Answer from the drawing. Dimensions are ordinates in mm from the lowest x, y and z of the part. A direction names the side the tool comes from. Round coordinates to 2 decimals unless told otherwise and drop trailing zeros. Write each loop counter-clockwise with the first axis right and the second up, starting at its lowest first coordinate (ties: lowest second). Pieces come first, ordered by that corner, then holes.
1. Find section A-A (y = 62). Write down the section's boundary in (x, z).
2. Find section C-C (z = 1.25). Write down the section's boundary in (x, y).
3. Find section D-D (x = 37). Write down the section's boundary in (y, z), and give its area (3 significant figures).
4. Flat-ended cylindrical pins translate along their axes: pin 1 Ø4 at (x, z) = (12.5, 4) entering from +Y (1 decimal); pin 2 Ø6 at (y, z) = (20.5, 8.5) entering from +X; pin 3 Ø2.5 at (x, y) = (46.9, 71.9) entering from -Z; pin 4 Ø5 at (x, z) = (4, 4) entering from +Y. Find the tip coordinate at first contact, or state that the pin passes through.
5. Find section B-B (x = 6). Write down the section's boundary in (y, z).
6. Straight lines are drawn through the part: probe 1 along X at (y, z) = (62.5, 4.75); probe 2 along Y at (x, z) = (37, 6.5); probe 3 along Y at (x, z) = (37, 2.05). For each, find the intervals that lie inside material, in ascending order.
7. A tool of negligible diameter and unlimited length cuts with its end or side. For the marked faces 1, 2 and 3, from which of +Z, -Z, +X, -X, +Y, -Y can it reach the whole face along a straight path? Write none if from no direction.
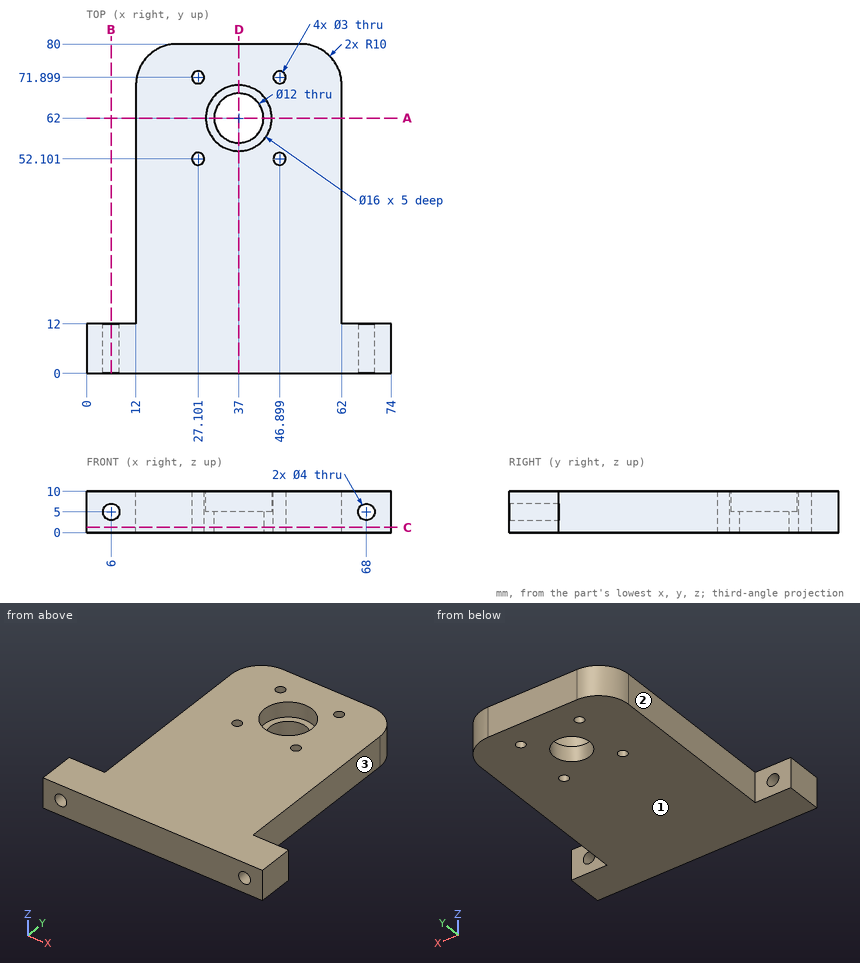
Worked answers:
1. outline: (12, 0) - (31, 0) - (31, 5) - (29, 5) - (29, 10) - (12, 10) - close; (43, 0) - (62, 0) - (62, 10) - (45, 10) - (45, 5) - (43, 5) - close
2. outline: (0, 0) - (74, 0) - (74, 12) - (62, 12) - (62, 70) arc R10 ccw to (52, 80) - (22, 80) arc R10 ccw to (12, 70) - (12, 12) - (0, 12) - close; hole circle Ø3 at (27.1, 52.1); hole circle Ø3 at (27.1, 71.9); hole circle Ø12 at (37, 62); hole circle Ø3 at (46.9, 52.1); hole circle Ø3 at (46.9, 71.9)
3. outline: (0, 0) - (56, 0) - (56, 5) - (54, 5) - (54, 10) - (0, 10) - close; (68, 0) - (80, 0) - (80, 10) - (70, 10) - (70, 5) - (68, 5) - close
3. area: 660 mm2
4. pin 1: stops at y = 76.6
4. pin 2: stops at x = 62
4. pin 3: passes through
4. pin 4: stops at y = 12
5. outline: (0, 0) - (12, 0) - (12, 3) - (0, 3) - close; (0, 7) - (12, 7) - (12, 10) - (0, 10) - close
6. probe 1: x = 12 to 31.02, 42.98 to 62
6. probe 2: y = 0 to 54, 70 to 80
6. probe 3: y = 0 to 56, 68 to 80
7. face 1: -Z, +X, -X, +Y, -Y
7. face 2: +Z, -Z, -X, +Y
7. face 3: +Z, -Z, +X, +Y
